Geometry check sheet. Reference: the model listing, model coordinates, mm. Coordinates: 2 decimals unless noted, no trailing zeros. Loops run counter-clockwise (first coordinate to the right, second up) from the corner with the lowest first, then second, coordinate; pieces in that order, holes last.
Autodesk Inventor part; units mm, degrees
ref_plane "YZ Plane" through (0, 0, 0) normal (1, 0, 0) x (0, 1, 0)
ref_plane "XZ Plane" through (0, 0, 0) normal (0, 1, 0) x (-1, 0, 0)
ref_plane "XY Plane" through (0, 0, 0) normal (0, 0, 1) x (1, 0, 0)
sketch "Sketch1" plane through (0, 0, 0) normal (0, 1, 0) x (-1, 0, 0)
  circle A0 centre (0, 0) radius 7
  dimension "d0" = 14
extrude "Extrusion1" add sketch "Sketch1" along normal blind 53
fillet "Fillet1" radius 2 2 edges at (7, 0, 0) (7, 53, 0)
ref_plane "Work Plane1" through (0, 15, 0) normal (0, -1, 0) x (1, 0, 0)
split_face "Split1"
properties part number "739136_AA"
1) Section check A-A on y = 43. Record the cut outline in (x, z), and give its area (3 significant figures).
Data:
outline: circle Ø14 at (0, 0)
area: 154 mm2
2) Depth check by flat-ended pin: pin 1 (1.5 mm diameter, centred on x = -4.5, z = -5, fed in from +Y); pin 2 (1.5 mm diameter, centred on y = 31.5, z = 5.5, fed in from -X); pin 3 (8 mm diameter, centred on y = 42.5, z = -4.5, fed in from +X). Enter the tip coordinate at first touch or a pass-through.
Data:
pin 1: stops at y = 52.75
pin 2: stops at x = -5.14
pin 3: stops at x = 6.98
3) Material ranges on probe 1 along Z at (x, y) = (-3, 9); probe 2 along Z at (x, y) = (-2, 33); probe 3 along X at (y, z) = (18, 3.5), recorded low to high.
Data:
probe 1: z = -6.32 to 6.32
probe 2: z = -6.71 to 6.71
probe 3: x = -6.06 to 6.06
